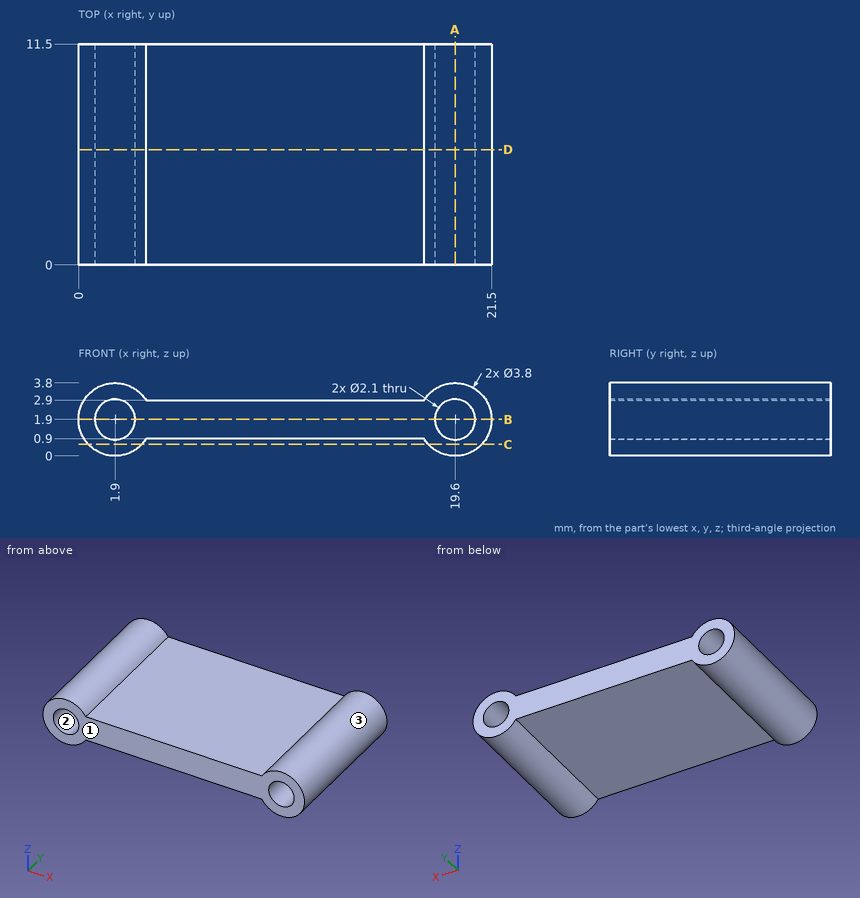
The figure shows three views and two pictorial views of one solid part (mm, origin at its lowest corner). Answer the questions. Give positions to 0.01 mm unless a question says otherwise; leave off trailing zeros. Loops run counter-clockwise (first coordinate to the right, second up) from the corner with the lowest first, then second, coordinate; pieces in that order, holes last. Notation, with made-up numbers: M -6.75,-19 L 38.25,-19 A27 cw 38.25,-1 Z; hole C 54,50.25 d7. An arc over 180 degrees is marked long. Write each question's results on one line, items separated by ' | '.
1. Section D-D on y = 6 is taken. Give the vertices of the cut face in (x, z), plus the area to 3 significant figures.
Values:
outline: M 3.52,0.9 L 17.98,0.9 A1.9 ccw long 17.98,2.9 L 3.52,2.9 A1.9 ccw long Z; hole C 1.9,1.9 d2.1; hole C 19.6,1.9 d2.1 | area: 43.9 mm^2
2. Given pin 1 (1 mm diameter, centred on x = 2.5, y = 3, fed in from -Z); pin 2 (1 mm diameter, centred on y = 7.5, z = 2.5, fed in from -X); pin 3 (1.3 mm diameter, centred on x = 1.9, z = 1.9, fed in from +Y); pin 4 (6 mm diameter, centred on x = 12.5, y = 3, fed in from +Z), each flat-ended and moving along its own axis, determine where each tip first touches the part or whether it passes through.
Values:
pin 1: stops at z = 0 | pin 2: stops at x = 0 | pin 3: passes through | pin 4: stops at z = 2.9
3. Section A-A on x = 19.6 is taken. Give the vertices of the cut face in (y, z).
Values:
outline: M 0,0 L 11.5,0 L 11.5,0.85 L 0,0.85 Z; M 0,2.95 L 11.5,2.95 L 11.5,3.8 L 0,3.8 Z
4. Section B-B on z = 1.9 is taken. Give the vertices of the cut face in (x, y).
Values:
outline: M 0,0 L 0.85,0 L 0.85,11.5 L 0,11.5 Z; M 2.95,0 L 18.55,0 L 18.55,11.5 L 2.95,11.5 Z; M 20.65,0 L 21.5,0 L 21.5,11.5 L 20.65,11.5 Z
5. Straight lines are drawn through the part: line 1 (X direction, y = 6.25, z = 2.4); line 2 (X direction, y = 2.25, z = 2.65) (3 decimals); line 3 (Z direction, x = 16.5, y = 4). For each, find the intervals that lie inside material, in ascending order. Write a range as [from, to].
Values:
line 1: x = [0.07, 0.98], [2.82, 18.68], [20.52, 21.43] | line 2: x = [0.154, 1.165], [2.635, 18.865], [20.335, 21.346] | line 3: z = [0.9, 2.9]
6. Section C-C on z = 0.6 is taken. Give the vertices of the cut face in (x, y).
Values:
outline: M 0.51,0 L 3.29,0 L 3.29,11.5 L 0.51,11.5 Z; M 18.21,0 L 20.99,0 L 20.99,11.5 L 18.21,11.5 Z
7. The mould has two halves that part along Z. Classify the marked faces 1, 2 and 3: pulls with the +Z half, pulls with the -Z half, needs draft (parallel to the pull), parting line crosses it, or undercut.
Values:
face 1: needs draft | face 2: undercut | face 3: parting line crosses it
